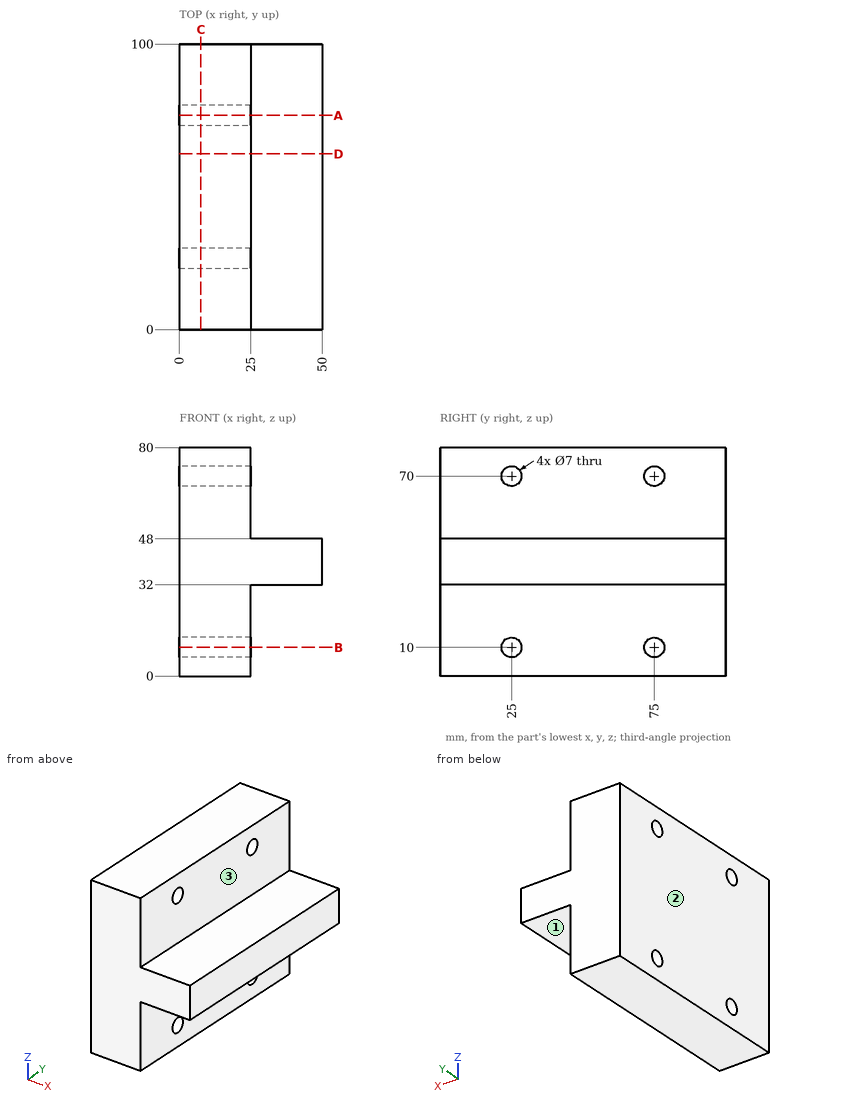
Study the drawing (mm; zero at the part's minimum x, y, z) and answer. A direction names the side the tool comes from. Give positions to 0.01 mm unless a question says otherwise; leave off trailing zeros. Write each loop counter-clockwise with the first axis right and the second up, starting at its lowest first coordinate (ties: lowest second). Pieces come first, ordered by that corner, then holes.
(1) The part is cut by section B-B on z = 10. Write down the section's boundary in (x, y), plus the area to 3 significant figures.
Final values:
outline: (0, 0) - (25, 0) - (25, 21.5) - (0, 21.5) - close; (0, 28.5) - (25, 28.5) - (25, 71.5) - (0, 71.5) - close; (0, 78.5) - (25, 78.5) - (25, 100) - (0, 100) - close
area: 2,150 mm2
(2) Flat-ended cylindrical pins translate along their axes: pin 1 Ø5.5 at (y, z) = (25, 70) entering from +X; pin 2 Ø16 at (y, z) = (52, 72) entering from +X; pin 3 Ø20 at (x, y) = (41, 60.5) entering from +Z. Find the tip coordinate at first contact, or state that the pin passes through.
Final values:
pin 1: passes through
pin 2: stops at x = 25
pin 3: stops at z = 48
(3) The part is cut by section C-C on x = 7.5. Write down the section's boundary in (y, z), plus the area to 3 significant figures.
Final values:
outline: (0, 0) - (100, 0) - (100, 80) - (0, 80) - close; hole circle Ø7 at (25, 10); hole circle Ø7 at (25, 70); hole circle Ø7 at (75, 10); hole circle Ø7 at (75, 70)
area: 7,850 mm2
(4) The part is cut by section A-A on y = 75. Write down the section's boundary in (x, z), plus the area to 3 significant figures.
Final values:
outline: (0, 0) - (25, 0) - (25, 6.5) - (0, 6.5) - close; (0, 13.5) - (25, 13.5) - (25, 32) - (50, 32) - (50, 48) - (25, 48) - (25, 66.5) - (0, 66.5) - close; (0, 73.5) - (25, 73.5) - (25, 80) - (0, 80) - close
area: 2,050 mm2
(5) Which of the six approach directions +Z, -Z, +X, -X, +Y, -Y give full straight-line access (tool end or side, diameter ignored) to the marked faces 1, 2 and 3?
Final values:
face 1: -Z, +X, +Y, -Y
face 2: +Z, -Z, -X, +Y, -Y
face 3: +Z, +X, +Y, -Y
(6) Straight lines are drawn through the part: line 1 (Z direction, x = 16, y = 25); line 2 (X direction, y = 85, z = 73); line 3 (Z direction, x = 30.5, y = 90). For each, find the intervals that lie inside material, in ascending order.
Final values:
line 1: z = 0 to 6.5, 13.5 to 66.5, 73.5 to 80
line 2: x = 0 to 25
line 3: z = 32 to 48
(7) The part is cut by section D-D on y = 61.5. Write down the section's boundary in (x, z), plus the area to 3 significant figures.
Final values:
outline: (0, 0) - (25, 0) - (25, 32) - (50, 32) - (50, 48) - (25, 48) - (25, 80) - (0, 80) - close
area: 2,400 mm2
